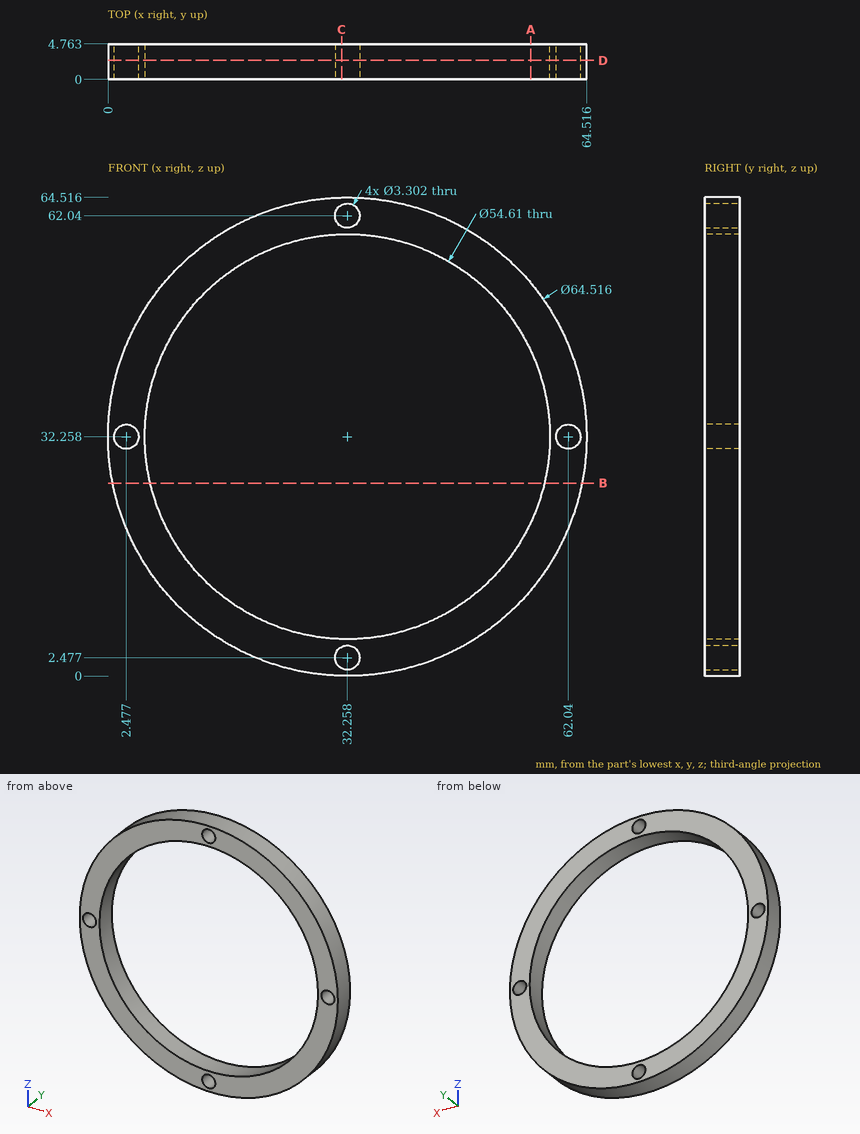
Study the drawing (mm; zero at the part's minimum x, y, z) and answer. Give positions to 0.01 mm unless a question says otherwise; leave off trailing zeros. Write each loop counter-clockwise with the first axis right and the second up, starting at its lowest first coordinate (ties: lowest second). Pieces come first, ordered by that corner, then holes. Notation, with made-up numbers: (-22, 48) -> (-3, 48) arc R26 cw to (-3, 74) -> close; hole circle Ø3 at (-15.75, 67). An arc over 180 degrees is marked (long way). Write item = value, one per line. Start each with the question number.
1) The part is cut by section D-D, the plane y = 2.55. Count the separate pieces of the cut face and the enclosed holes in it.
2) The part is cut by section A-A, the plane x = 57. Determine the outline of the cut face in (y, z).
3) Straight lines are drawn through the part: line 1 along Z through (x, y) = (31.5, 3.85) (1 decimal); line 2 along Z through (x, y) = (35.5, 4.35) (1 decimal); line 3 along X through (y, z) = (4.65, 53.5) (1 decimal). For each, find the intervals that lie inside material, in ascending order.
4) The part is cut by section C-C, the plane x = 31.5. Determine the outline of the cut face in (y, z).
5) The part is cut by section B-B, the plane z = 26. Determine the outline of the cut face in (x, y).
6) Each of these flat-tipped pins is pushed along its axis until it touches: pin 1 (2 mm diameter, centred on x = 10, y = 2.5, fed in from -Z) (1 decimal); pin 2 (1.5 mm diameter, centred on x = 46, y = 2.5, fed in from +Z) (1 decimal); pin 3 (2 mm diameter, centred on x = 12.5, y = 1, fed in from +Z). Where does it stop, or does it pass through?
Solutions:
q1.separate_pieces = 1
q1.enclosed_holes = 5
q2.outline = (0, 11.56) -> (4.76, 11.56) -> (4.76, 20.71) -> (0, 20.71) -> close; (0, 43.81) -> (4.76, 43.81) -> (4.76, 52.96) -> (0, 52.96) -> close
q3.line_1 = 0 to 1, 3.9 to 5, 59.6 to 60.6, 63.5 to 64.5
q3.line_2 = 0.2 to 5.1, 59.4 to 64.4
q3.line_3 = 8 to 15.1, 49.4 to 56.5
q4.outline = (0, 0.01) -> (4.76, 0.01) -> (4.76, 1.01) -> (0, 1.01) -> close; (0, 3.94) -> (4.76, 3.94) -> (4.76, 4.96) -> (0, 4.96) -> close; (0, 59.55) -> (4.76, 59.55) -> (4.76, 60.57) -> (0, 60.57) -> close; (0, 63.51) -> (4.76, 63.51) -> (4.76, 64.51) -> (0, 64.51) -> close
q5.outline = (0.61, 0) -> (5.68, 0) -> (5.68, 4.76) -> (0.61, 4.76) -> close; (58.84, 0) -> (63.9, 0) -> (63.9, 4.76) -> (58.84, 4.76) -> close
q6.pin_1 = 8
q6.pin_2 = 61.8
q6.pin_3 = 58.5
